Autodesk Inventor part; units mm, degrees
ref_plane "YZ Plane" through (0, 0, 0) normal (1, 0, 0) x (0, 1, 0)
ref_plane "XZ Plane" through (0, 0, 0) normal (0, 1, 0) x (-1, 0, 0)
ref_plane "XY Plane" through (0, 0, 0) normal (0, 0, 1) x (1, 0, 0)
sketch "Sketch15" plane through (0, 0, 0) normal (0, 1, 0) x (-1, 0, 0)
  circle A0 centre (0, 0) radius 2.75
  circle A1 centre (0, 0) radius 5
  line L0 (0, 0) -> (0, -28)
  line L1 (0, -33) -> (0, -23) construction
  line L2 (2.75, -33) -> (2.75, -23)
  line L3 (-2.75, -23) -> (-2.75, -33)
  arc A2 (-2.75, -33) -> (2.75, -33) centre (0, -33) ccw
  arc A3 (2.75, -23) -> (-2.75, -23) centre (0, -23) ccw
  line L4 (0, -43) -> (0, -13) construction
  line L5 (0, 0) -> (0, -14)
  line L6 (-5.5, -15.5) -> (5.5, -15.5)
  line L7 (5.5, -15.5) -> (5.5, -10.5)
  line L8 (5.5, -10.5) -> (-5.5, -10.5)
  line L9 (-5.5, -10.5) -> (-5.5, -15.5)
  line L10 (-5.5, -15.5) -> (5.5, -10.5) construction
  line L11 (5.5, -15.5) -> (-5.5, -10.5) construction
  line L12 (5, 0) -> (5.5, -10.5)
  line L13 (-5, 0) -> (-5.5, -10.5)
  line L14 (0, -35.75) -> (0, -20.25) construction
  line L15 (5, -35.75) -> (5, -20.25)
  line L16 (-5, -20.25) -> (-5, -35.75)
  arc A4 (-5, -35.75) -> (5, -35.75) centre (0, -35.75) ccw
  arc A5 (5, -20.25) -> (-5, -20.25) centre (0, -20.25) ccw
  line L17 (5.5, -15.5) -> (5, -20.25)
  line L18 (-5.5, -15.5) -> (-5, -20.25)
  line L19 (0, 0) -> (0, 25)
  circle A6 centre (0, 25) radius 2.75
  circle A7 centre (0, 25) radius 5
  line L20 (0, 25) -> (5, 25)
  line L21 (0, 25) -> (-5, 25)
  line L22 (5, 25) -> (5, 0)
  line L23 (-5, 25) -> (-5, 0)
  point P0 (-1.5612, -15.5)
  point P1 (1.5612, -15.5)
  dimension "d102" = 5.5
  dimension "d103" = 10
  dimension "d104" = 28
  dimension "d105" = 5
  dimension "d106" = 5.5
  dimension "d107" = 15
  dimension "d109" = 14
  dimension "d110" = 11
  dimension "d111" = 5
  dimension "d112" = 10
  dimension "d133" = 25
  dimension "d134" = 5.5
  dimension "d135" = 10
extrude "Extrusion14" add sketch "Sketch15" along normal blind 1 contours A0 L19 A1 L0 | A0 L0 A1 L19 | L19 A7 L22 A1 | A1 L23 A7 L19 | L0 L8 L13 A1 | A1 L12 L8 L0 | A7 L21 A6 L19 | L19 A6 L20 A7 | L8 L7 L6 A5 L0 | L0 A5 L6 L9 L8 | L20 A6 L21 A7 | L17 A5 L6 | L6 A5 L18 | A5 L6 L0 | L0 L6 A5 | A5 L15 A4 L16 L6
sketch "Sketch16" plane through (0, 1, 0) normal (0, 1, 0) x (1, 0, 0)
  circle A0 centre (0, 0) radius 2.75
  circle A1 centre (0, 0) radius 2.75
  arc A2 (-5, 0) -> (5, 0) centre (0, 0) ccw
  circle A3 centre (0, 0) radius 5
  line L0 (-2.75, 23) -> (-2.75, 33)
  line L1 (-2.75, 28) -> (0, 28)
  line L2 (0, 33) -> (0, 23) construction
  line L3 (-2.75, 33) -> (-2.75, 23)
  line L4 (2.75, 23) -> (2.75, 33)
  arc A4 (2.75, 33) -> (-2.75, 33) centre (0, 33) ccw
  arc A5 (-2.75, 23) -> (2.75, 23) centre (0, 23) ccw
  line L5 (0, 33) -> (0, 23) construction
  line L6 (-4, 33) -> (-4, 23)
  line L7 (4, 23) -> (4, 33)
  arc A6 (4, 33) -> (-4, 33) centre (0, 33) ccw
  arc A7 (-4, 23) -> (4, 23) centre (0, 23) ccw
  circle A8 centre (0, -25) radius 2.75
  circle A9 centre (0, -25) radius 2.75
  circle A10 centre (0, -25) radius 5
  point P0 (5, 0)
  dimension "d115" = 5
  dimension "d116" = 5.5
  dimension "d117" = 5
  dimension "d118" = 8
  dimension "d136" = 5.5
  dimension "d137" = 10
extrude "Extrusion15" add sketch "Sketch16" along normal blind 2
sketch "Sketch17" plane through (0, 1, 0) normal (0, 1, 0) x (1, 0, 0)
  line L0 (0, 0) -> (0, 13)
  line L1 (5.5, 16) -> (-5.5, 16)
  line L2 (-5.5, 16) -> (-5.5, 10)
  line L3 (-5.5, 10) -> (5.5, 10)
  line L4 (5.5, 10) -> (5.5, 16)
  line L5 (5.5, 16) -> (-5.5, 10) construction
  line L6 (-5.5, 16) -> (5.5, 10) construction
  dimension "d121" = 13
  dimension "d129" = 11
  dimension "d130" = 6
extrude "Extrusion16" add sketch "Sketch17" along normal blind 2
fillet "Fillet7" radius 1 4 edges at (-5.5, 2, -10) (-5.5, 2, -16) (5.5, 2, -10) (5.5, 2, -16)
fillet "Fillet8" radius 1 8 edges at (5.2071, 3, -10.2929) (5.5, 3, -13) (5.2071, 3, -15.7071) (0, 3, -16) (-5.2071, 3, -15.7071) (-5.5, 3, -13) (-5.2071, 3, -10.2929) (0, 3, -10)
properties part number "Belt_Restraint"
The listing builds one solid part. Answer for the finished solid, in the listing's coordinates (mm). A direction names the side the tool comes from. Give positions to 0.01 mm unless a question says otherwise; leave off trailing zeros. Write each loop counter-clockwise with the first axis right and the second up, starting at its lowest first coordinate (ties: lowest second). Pieces come first, ordered by that corner, then holes.
Item 1: Flat-ended cylindrical pins translate along their axes: P1, Ø1, axis at y = 2, z = -30, coming from the +X side; P2, Ø0.5, axis at x = 2, y = 1.5, coming from the +Z side; P3, Ø1.5, axis at y = 0.5, z = 3, coming from the +X side. Find the tip coordinate at first contact, or state that the pin passes through.
Item 2: Find the intervals of material crossed by line 1 along Z through (x, y) = (-0.75, 0.6); line 2 along X through (y, z) = (1.85, 0); line 3 along Z through (x, y) = (-2, 0.4), in increasing order.
Item 3: Section A-A, the plane z = -29 is taken. Write down the section's boundary in (x, y).
Item 4: Which of the six approach directions +Z, -Z, +X, -X, +Y, -Y give full straight-line access (tool end or side, diameter ignored) to faces 5 (the flat face through (-4.8, 1, -25.2)), 6 (the flat face through (4, 2, -28)), 7 (the flat face through (-4, 2, -28))?
Item 5: Section C-C, the plane y = 0.45 is taken. Write down the section's boundary in (x, z).
Item 6: Determine the mould class of faces 1 (the cylindrical face through (0.06, 1.48, -20.25)), 2 (the flat face through (0, 1, 13)), 3 (the flat face through (0, 3, -13)), 4 (the cylindrical face through (0, 2, -37)) for opening direction Z: released by +Z, released by -Z, zero draft, split by the parting line, or undercut.
Completed:
1. P1: stops at x = 4
1. P2: stops at z = 29.68
1. P3: stops at x = 5
2. line 1: z = -40.69 to -35.65, -20.35 to -2.65, 2.65 to 22.35, 27.65 to 29.94
2. line 2: x = -5 to -2.75, 2.75 to 5
2. line 3: z = -40.33 to -34.89, -21.11 to -1.89, 1.89 to 23.11, 26.89 to 29.58
3. outline: (-5, 0) - (-2.75, 0) - (-2.75, 3) - (-4, 3) - (-4, 1) - (-5, 1) - close; (2.75, 0) - (5, 0) - (5, 1) - (4, 1) - (4, 3) - (2.75, 3) - close
4. face 5: +Y
4. face 6: -Z, +X, +Y
4. face 7: -Z, -X, +Y
5. outline: (-5.5, -15.5) - (-5, -20.25) - (-5, -35.75) arc R5 ccw to (5, -35.75) - (5, -20.25) - (5.5, -15.5) - (5.5, -10.5) - (5, 0) - (5, 25) arc R5 ccw to (-5, 25) - (-5, 0) - (-5.5, -10.5) - close; hole (-2.75, -33) arc R2.75 ccw to (2.75, -33) - (2.75, -23) arc R2.75 ccw to (-2.75, -23) - close; hole circle Ø5.5 at (0, 0); hole circle Ø5.5 at (0, 25)
6. face 1: undercut
6. face 2: undercut
6. face 3: zero draft
6. face 4: released by -Z
